Part model, mm, in its own coordinate system. A direction names the side the tool comes from. Coordinates: 2 decimals unless noted, no trailing zeros. Write each loop counter-clockwise with the first axis right and the second up, starting at its lowest first coordinate (ties: lowest second). Pieces come first, ordered by that corner, then holes. Notation, with made-up numbers: M 69,87 L 102,87 A24 ccw 102,118 Z; hole C 66,-39.75 d8. An arc over 180 degrees is marked long. Use a Markdown table: item, result. Add a question column.
Q1. Wall check: L1, parallel to X at y = 37.5, z = 0.75; L2, parallel to X at y = 23, z = 4.25; L3, parallel to Y at x = 45.5, z = 2. Give the ranges that are in metal, low to high. Write a range as from..to.
Q2. Slice it at C-C on z = 1.5. Write the cut outline in (x, y), then the cut area to 3 significant figures.
Q3. Slice it at A-A on x = 29.5. Write the cut outline in (y, z).
Q4. Tool access for faces 4 (the flat face through (1, 27, 6)), 5 (the flat face through (44.8, -2, 5)), 6 (the flat face through (0, 27, 4)): list every direction of +Z, -Z, +X, -X, +Y, -Y with a clear straight run to the whole face (end or side of a thin tool).
Q5. Slice it at B-B on y = 11. Write the cut outline in (x, z).
Q6. Mould opens along Y. For faces 1 (the flat face through (32, 1.5, 1)), 2 (the flat face through (30, -1, 3)), 3 (the flat face through (66, 30, 6)) say: released by +Y, released by -Y, zero draft, split by the parting line, or undercut.
Q7. Slice it at D-D on x = 2.5. Write the cut outline in (y, z).
Q8. Pin check, flat tips, straight feed: pin 1 Ø4.5 at (x, y) = (17, 55.5) entering from +Z; pin 2 Ø3 at (x, z) = (54, 4) entering from +Y; pin 3 Ø2 at (x, y) = (66.5, 38.5) entering from +Z. Stop position of each tip, or through.
from build123d import *

# Parameters (mm, degrees)
BOX004_W      = 4
BOX004_H      = 55
BOX004_DEPTH  = 2
BOX005_W      = 4
BOX005_H      = 55
BOX005_DEPTH  = 2
BOX006_W      = 5
BOX006_H      = 30
BOX006_DEPTH  = 1.5
BOX007_W      = 24
BOX007_H      = 4
BOX007_DEPTH  = 3.5
BOX010_W      = 8
BOX010_H      = 4
BOX010_DEPTH  = 3.5
BOX003_W      = 5
BOX003_H      = 55
BOX003_DEPTH  = 1.5
BOX011_W      = 5.5
BOX011_H      = 59
BOX011_DEPTH  = 3
BOX012_W      = 5.5
BOX012_H      = 59
BOX012_DEPTH  = 3
BOX013_W      = 68.8
BOX013_H      = 5.5
BOX013_DEPTH  = 3
SKETCH003_W   = 72.8
SKETCH003_H   = 63
SKETCH003_W_2 = 61.8
SKETCH003_H_2 = 52
PAD003_DEPTH  = 1.5


with BuildPart() as middle_pad:
    # Box004 → Box004 (new body)
    with BuildSketch(Plane(origin=(-4, 0, 0), x_dir=(1, 0, 0), z_dir=(0, 0, 1))):
        with Locations((2, 27.5)):
            Rectangle(BOX004_W, BOX004_H)
    extrude(amount=BOX004_DEPTH)


with BuildPart() as middle_pad001:
    # Box005 → Box005 (new body)
    with BuildSketch(Plane(origin=(64.8, 0, 0), x_dir=(1, 0, 0), z_dir=(0, 0, 1))):
        with Locations((2, 27.5)):
            Rectangle(BOX005_W, BOX005_H)
    extrude(amount=BOX005_DEPTH)


with BuildPart() as top_cover001:
    # Box006 → Box006 (new body)
    with BuildSketch(Plane(origin=(63.8, 0, 2), x_dir=(1, 0, 0), z_dir=(0, 0, 1))):
        with Locations((2.5, 15)):
            Rectangle(BOX006_W, BOX006_H)
    extrude(amount=BOX006_DEPTH)


with BuildPart() as middle_pad002:
    # Box007 → Box007 (new body)
    with BuildSketch(Plane(origin=(44.8, -4, 0), x_dir=(1, 0, 0), z_dir=(0, 0, 1))):
        with Locations((12, 2)):
            Rectangle(BOX007_W, BOX007_H)
    extrude(amount=BOX007_DEPTH)


with BuildPart() as side_pad:
    # Box010 → Box010 (new body)
    with BuildSketch(Plane(origin=(-4, -4, 0), x_dir=(1, 0, 0), z_dir=(0, 0, 1))):
        with Locations((4, 2)):
            Rectangle(BOX010_W, BOX010_H)
    extrude(amount=BOX010_DEPTH)


with BuildPart() as fusion002:
    # Box003 → Box003 (new body)
    with BuildSketch(Plane(origin=(-4, 0, 2), x_dir=(1, 0, 0), z_dir=(0, 0, 1))):
        with Locations((2.5, 27.5)):
            Rectangle(BOX003_W, BOX003_H)
    extrude(amount=BOX003_DEPTH)

    # Fusion002: union middle_pad, middle_pad001, top cover001, middle_pad002, side_pad
    add(middle_pad.part)
    add(middle_pad001.part)
    add(top_cover001.part)
    add(middle_pad002.part)
    add(side_pad.part)


with BuildPart() as fusion002_1:
    # Fusion002 placement: moved
    add(fusion002.part.moved(Location((0, 0, 3))))


with BuildPart() as cube003:
    # Box011 → Box011 (new body)
    with BuildSketch(Plane(origin=(-4, -4, 0), x_dir=(1, 0, 0), z_dir=(0, 0, 1))):
        with Locations((2.75, 29.5)):
            Rectangle(BOX011_W, BOX011_H)
    extrude(amount=BOX011_DEPTH)


with BuildPart() as cube004:
    # Box012 → Box012 (new body)
    with BuildSketch(Plane(origin=(63.3, -4, 0), x_dir=(1, 0, 0), z_dir=(0, 0, 1))):
        with Locations((2.75, 29.5)):
            Rectangle(BOX012_W, BOX012_H)
    extrude(amount=BOX012_DEPTH)


with BuildPart() as cube005:
    # Box013 → Box013 (new body)
    with BuildSketch(Plane(origin=(-1.5, -4, 0), x_dir=(1, 0, 0), z_dir=(0, 0, 1))):
        with Locations((34.4, 2.75)):
            Rectangle(BOX013_W, BOX013_H)
    extrude(amount=BOX013_DEPTH)


with BuildPart() as fusion001:
    # Sketch003 → Pad003 (new body)
    with BuildSketch(Plane.XY):
        with Locations((32.4, 27.5)):
            Rectangle(SKETCH003_W, SKETCH003_H)
        with Locations((32.4, 27.5)):
            Rectangle(SKETCH003_W_2, SKETCH003_H_2, mode=Mode.SUBTRACT)
    extrude(amount=-PAD003_DEPTH)

    # Fusion001: union Fusion002, Cube003, Cube004, Cube005
    add(fusion002_1.part)
    add(cube003.part)
    add(cube004.part)
    add(cube005.part)


solid = fusion001.part
Recorded:
| question | item | result |
|---|---|---|
| 1 | L1 | -4..1.5, 63.3..68.8 |
| 1 | L2 | -4..0, 64.8..68.8 |
| 1 | L3 | -4..1.5 |
| 2 | outline | M -4,-4 L 68.8,-4 L 68.8,55 L 63.3,55 L 63.3,1.5 L 1.5,1.5 L 1.5,55 L -4,55 Z |
| 2 | area | 989 mm² |
| 3 | outline | M -4,-1.5 L 1.5,-1.5 L 1.5,3 L -4,3 Z; M 53.5,-1.5 L 59,-1.5 L 59,0 L 53.5,0 Z |
| 4 | face 4 | +Z, +Y |
| 4 | face 5 | +Z, +Y, -Y |
| 4 | face 6 | +Y |
| 5 | outline | M -4,-1.5 L 1.5,-1.5 L 1.5,3 L 0,3 L 0,5 L 1,5 L 1,6.5 L -4,6.5 Z; M 63.3,-1.5 L 68.8,-1.5 L 68.8,6.5 L 63.8,6.5 L 63.8,5 L 64.8,5 L 64.8,3 L 63.3,3 Z |
| 6 | face 1 | undercut |
| 6 | face 2 | zero draft |
| 6 | face 3 | released by +Y |
| 7 | outline | M -4,-1.5 L 1.5,-1.5 L 1.5,3 L 0,3 L 0,6.5 L -4,6.5 Z; M 53.5,-1.5 L 59,-1.5 L 59,0 L 53.5,0 Z |
| 8 | pin 1 | z = 0 |
| 8 | pin 2 | y = 1.5 |
| 8 | pin 3 | z = 5 |
